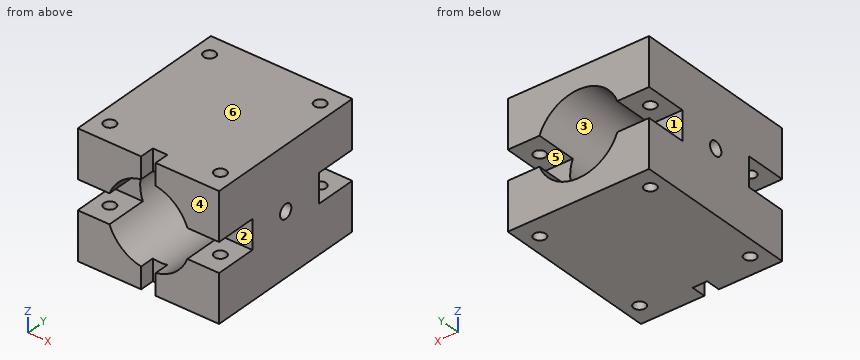
```python
from build123d import *

# Parameters (mm, degrees)
SKETCH1_R                       = 20
BOSS_EXTRUDE1_DEPTH             = 40
SKETCH26_W                      = 0.434993995
SKETCH26_H                      = 14
CUT_EXTRUDE19_DEPTH             = 20
SKETCH30_W                      = 92.939365228
SKETCH30_H                      = 14
CUT_EXTRUDE22_DEPTH             = 20
CUT_EXTRUDE20_REACH             = 62.465
SKETCH27_R                      = 2.830219018
CUT_EXTRUDE20_DIRECTION_2_REACH = 62.465
CUT_EXTRUDE24_START             = -20
SKETCH33_R                      = 3.4
CUT_EXTRUDE24_DEPTH             = 50
SKETCH37_W                      = 7
SKETCH37_H                      = 70.017745432
CUT_EXTRUDE26_DEPTH             = 7


with BuildPart() as part:
    # Sketch1 → Boss-Extrude1 (new, symmetric)
    with BuildSketch(Plane(origin=(0, 0, 0), x_dir=(1, 0, 0), z_dir=(0, 1, 0))):
        Polygon((-20, -30), (34, -30), (34, 30), (-20, 30), (-34, 30), (-34, -30), align=None)
        with Locations(Location((0, 0, 0), (0, 0, 270))):
            Circle(SKETCH1_R, mode=Mode.SUBTRACT)
    extrude(amount=BOSS_EXTRUDE1_DEPTH, both=True)

    # Sketch26 → Cut-Extrude19 (cut)
    with BuildSketch(Plane(origin=(0, 40, 0), x_dir=(1, 0, 0), z_dir=(0, 1, 0))):
        with BuildLine():
            ThreePointArc((20, 0), (19.681207787, -3.55669229), (18.734993995, -7))
            Line((18.734993995, -7), (34, -7))
            Line((34, -7), (34, 7))
            Line((34, 7), (18.734993995, 7))
            ThreePointArc((18.734993995, 7), (19.681207787, 3.55669229), (20, 0))
        make_face()
        with Locations((34.217496997, 0)):
            Rectangle(SKETCH26_W, SKETCH26_H)
        with BuildLine():
            Line((18.734993995, 7), (18.734993995, -7))
            ThreePointArc((18.734993995, -7), (19.681207787, -3.55669229), (20, 0))
            ThreePointArc((20, 0), (19.681207787, 3.55669229), (18.734993995, 7))
        make_face()
        with BuildLine():
            Line((-34, -7), (-18.734993995, -7))
            ThreePointArc((-18.734993995, -7), (-20, 0), (-18.734993995, 7))
            Line((-18.734993995, 7), (-34, 7))
            Line((-34, 7), (-34, -7))
        make_face()
    extrude(amount=-CUT_EXTRUDE19_DEPTH, mode=Mode.SUBTRACT)

    # Sketch30 → Cut-Extrude22 (cut)
    with BuildSketch(Plane.XZ.offset(40)):
        Rectangle(SKETCH30_W, SKETCH30_H)
    extrude(amount=-CUT_EXTRUDE22_DEPTH, mode=Mode.SUBTRACT)

    # Cut-Extrude20: up to this face of the body (flat: up to its plane)
    cut_extrude20_end = Plane(part.part.faces().sort_by_distance((0, 0, 30))[0])
    # Sketch27 → Cut-Extrude20 (cut, up to the picked face)
    with BuildSketch(Plane(origin=(0, 0, 0), x_dir=(-1, 0, 0), z_dir=(0, 0, -1)), mode=Mode.PRIVATE) as cut_extrude20_sk1:
        with Locations((26.58, 30)):
            Circle(SKETCH27_R)
    cut_extrude20_tool1 = split(extrude(cut_extrude20_sk1.sketch, amount=-CUT_EXTRUDE20_REACH, mode=Mode.PRIVATE), bisect_by=cut_extrude20_end, keep=Keep.BOTH, mode=Mode.PRIVATE)
    # Sketch27 → Cut-Extrude20 (cut, up to the picked face)
    with BuildSketch(Plane(origin=(0, 0, 0), x_dir=(-1, 0, 0), z_dir=(0, 0, -1)), mode=Mode.PRIVATE) as cut_extrude20_sk2:
        with Locations((-26.58, 30)):
            Circle(SKETCH27_R)
    cut_extrude20_tool2 = split(extrude(cut_extrude20_sk2.sketch, amount=-CUT_EXTRUDE20_REACH, mode=Mode.PRIVATE), bisect_by=cut_extrude20_end, keep=Keep.BOTH, mode=Mode.PRIVATE)
    cut_extrude20_1 = cut_extrude20_tool1.solids().sort_by(Axis((-26.58, 30, 0), (0, 0, 1)))[0]
    add(cut_extrude20_1, mode=Mode.SUBTRACT)
    cut_extrude20_2 = cut_extrude20_tool2.solids().sort_by(Axis((26.58, 30, 0), (0, 0, 1)))[0]
    add(cut_extrude20_2, mode=Mode.SUBTRACT)
    cut_extrude20 = cut_extrude20_1 + cut_extrude20_2  # Cut-Extrude20 as one shape, for the pattern or mirror that repeats it

    # Cut-Extrude20 direction 2: up to this face of the body (flat: up to its plane)
    cut_extrude20_direction_2_end = Plane(part.part.faces().sort_by_distance((0, 0, -30))[0])
    # Sketch27 → Cut-Extrude20 direction 2 (cut, up to the picked face)
    with BuildSketch(Plane(origin=(0, 0, 0), x_dir=(-1, 0, 0), z_dir=(0, 0, -1)), mode=Mode.PRIVATE) as cut_extrude20_direction_2_sk1:
        with Locations((26.58, 30)):
            Circle(SKETCH27_R)
    cut_extrude20_direction_2_tool1 = split(extrude(cut_extrude20_direction_2_sk1.sketch, amount=CUT_EXTRUDE20_DIRECTION_2_REACH, mode=Mode.PRIVATE), bisect_by=cut_extrude20_direction_2_end, keep=Keep.BOTH, mode=Mode.PRIVATE)
    # Sketch27 → Cut-Extrude20 direction 2 (cut, up to the picked face)
    with BuildSketch(Plane(origin=(0, 0, 0), x_dir=(-1, 0, 0), z_dir=(0, 0, -1)), mode=Mode.PRIVATE) as cut_extrude20_direction_2_sk2:
        with Locations((-26.58, 30)):
            Circle(SKETCH27_R)
    cut_extrude20_direction_2_tool2 = split(extrude(cut_extrude20_direction_2_sk2.sketch, amount=CUT_EXTRUDE20_DIRECTION_2_REACH, mode=Mode.PRIVATE), bisect_by=cut_extrude20_direction_2_end, keep=Keep.BOTH, mode=Mode.PRIVATE)
    cut_extrude20_direction_2_1 = cut_extrude20_direction_2_tool1.solids().sort_by(Axis((-26.58, 30, 0), (0, 0, -1)))[0]
    add(cut_extrude20_direction_2_1, mode=Mode.SUBTRACT)
    cut_extrude20_direction_2_2 = cut_extrude20_direction_2_tool2.solids().sort_by(Axis((26.58, 30, 0), (0, 0, -1)))[0]
    add(cut_extrude20_direction_2_2, mode=Mode.SUBTRACT)
    cut_extrude20_direction_2 = cut_extrude20_direction_2_1 + cut_extrude20_direction_2_2  # Cut-Extrude20 direction 2 as one shape, for the pattern or mirror that repeats it

    # Mirror1: Cut-Extrude20, Cut-Extrude20 direction 2 across plane
    add(cut_extrude20.mirror(Plane.ZX), mode=Mode.SUBTRACT)
    add(cut_extrude20_direction_2.mirror(Plane.ZX), mode=Mode.SUBTRACT)

    # Sketch33 → Cut-Extrude24 (cut)
    with BuildSketch(Plane.ZY.offset(34).offset(CUT_EXTRUDE24_START)):
        with Locations(Location((0, 0, 0), (0, 0, 180))):
            Circle(SKETCH33_R)
    cut_extrude24 = extrude(amount=CUT_EXTRUDE24_DEPTH, mode=Mode.SUBTRACT)

    # Mirror6: Cut-Extrude24 across plane
    add(cut_extrude24.mirror(Plane(origin=(0, 0, 0), x_dir=(0, 0, 1), z_dir=(1, 0, 0))), mode=Mode.SUBTRACT)

    # Sketch37 → Cut-Extrude26 (cut)
    with BuildSketch(Plane.XZ.offset(40)):
        Rectangle(SKETCH37_W, SKETCH37_H)
    extrude(amount=-CUT_EXTRUDE26_DEPTH, mode=Mode.SUBTRACT)


solid = part.part
```
The model under review builds one solid part; all positions refer to its coordinate system, in mm. Face numbers are marked on the shaded views. A direction names the side the tool comes from. Round coordinates to 2 decimals unless told otherwise and drop trailing zeros. Loops run counter-clockwise (first coordinate to the right, second up) from the corner with the lowest first, then second, coordinate; pieces in that order, holes last.
Item 1: For line 1 (Y direction, x = -26.58, z = -14); line 2 (X direction, y = 30, z = -24.25); line 3 (Y direction, x = 29, z = 0), list the stretches that pass through material, from the lowest coordinate up.
Determined:
line 1: y = -40 to -32.83, -27.17 to 27.17, 32.83 to 40
line 2: x = -34 to -29.41, -23.75 to 23.75, 29.41 to 34
line 3: y = -20 to -3.4, 3.4 to 20
Item 2: Take a section at D-D (z = 0). Write out the cut boundary in (x, y).
Determined:
outline: (-34, -20) - (-20, -20) - (-20, -3.4) - (-34, -3.4) - close; (-34, 3.4) - (-20, 3.4) - (-20, 20) - (-34, 20) - close; (20, -20) - (34, -20) - (34, -3.4) - (20, -3.4) - close; (20, 3.4) - (34, 3.4) - (34, 20) - (20, 20) - close
Item 3: Take a section at C-C (z = -13.5). Write out the cut boundary in (x, y), then the cut area to 3 significant figures.
Determined:
outline: (-34, -40) - (-14.76, -40) - (-14.76, 40) - (-34, 40) - close; (14.76, -40) - (34, -40) - (34, 40) - (14.76, 40) - close; hole circle Ø5.66 at (-26.58, -30); hole circle Ø5.66 at (-26.58, 30); hole circle Ø5.66 at (26.58, -30); hole circle Ø5.66 at (26.58, 30)
area: 2,980 mm2
Item 4: Take a section at A-A (y = 0). Write out the cut boundary in (x, z), then the cut area to 3 significant figures.
Determined:
outline: (-34, -30) - (34, -30) - (34, -3.4) - (19.71, -3.4) arc R20 cw to (-19.71, -3.4) - (-34, -3.4) - close; (-34, 3.4) - (-19.71, 3.4) arc R20 cw to (19.71, 3.4) - (34, 3.4) - (34, 30) - (-34, 30) - close
area: 2,630 mm2
Item 5: Clearance check with a flat-ended pin moving along its axis: pin 1 Ø2 at (x, z) = (0, -25.5) entering from -Y. State where the tip first meets the part, or that it passes through.
Determined:
pin 1: stops at y = -33
Item 6: Mouldability with a two-part tool opening along Z and no side actions: class the marked faces 4, 5 and 6 as released by +Z, released by -Z, zero draft, split by the parting line, or undercut.
Determined:
face 4: zero draft
face 5: undercut
face 6: released by +Z
Item 7: For the marked faces 1, 2 and 3, list the 3-axis set-ups (+Z, -Z, +X, -X, +Y, -Y) from which the entire face can be reached by the end or side of a thin tool; tool diameter is ignored.
Determined:
face 1: +X, -X, +Y
face 2: +X, -X, -Y
face 3: +Y, -Y
Item 8: Take a section at B-B (x = -26.58). Give the number of separate pieces and of enclosed holes in the cut face, then the cut area to 3 significant figures.
Determined:
separate pieces: 5
enclosed holes: 1
area: 3,680 mm2
